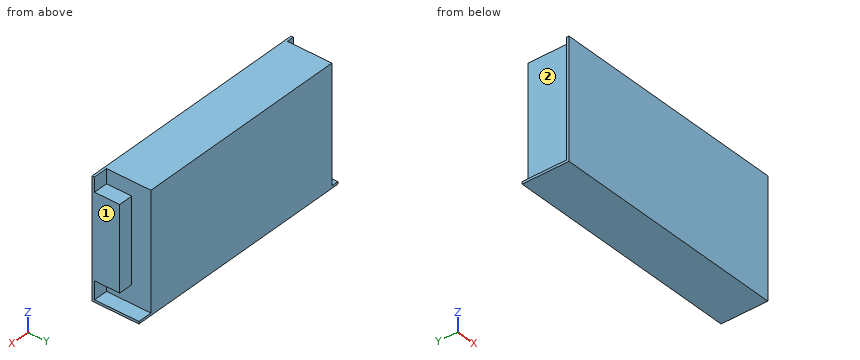
from build123d import *

# Parameters (mm, degrees)
SKETCH_1_W          = 199
SKETCH_1_H          = 99
EXTRUDE_1_DEPTH     = 39
SKETCH_2_W          = 6
SKETCH_2_H          = 97
SKETCH_2_W_2        = 12
CUT_EXTRUDE_1_DEPTH = 37
SKETCH_3_W          = 70
SKETCH_3_H          = 23
EXTRUDE_2_DEPTH     = 12


with BuildPart() as part:
    # Эскиз1 → Бобышка-Вытянуть1 (new body)
    with BuildSketch(Plane(origin=(0, 0, 0), x_dir=(1, 0, 0), z_dir=(0, 1, 0))):
        with Locations((99.5, 49.5)):
            Rectangle(SKETCH_1_W, SKETCH_1_H)
    extrude(amount=EXTRUDE_1_DEPTH)

    # Эскиз2 → Вырез-Вытянуть1 (cut)
    with BuildSketch(Plane(origin=(0, 39, 0), x_dir=(1, 0, 0), z_dir=(0, 1, 0))):
        with Locations((3, 48.5)):
            Rectangle(SKETCH_2_W, SKETCH_2_H)
        with Locations((193, 48.5)):
            Rectangle(SKETCH_2_W_2, SKETCH_2_H)
    extrude(amount=-CUT_EXTRUDE_1_DEPTH, mode=Mode.SUBTRACT)

    # Эскиз3 → Бобышка-Вытянуть2 (add)
    with BuildSketch(Plane(origin=(187, 0, 0), x_dir=(0, 0, -1), z_dir=(1, 0, 0))):
        with Locations((47, 11.5)):
            Rectangle(SKETCH_3_W, SKETCH_3_H)
    extrude(amount=EXTRUDE_2_DEPTH)


solid = part.part
Verification items for the finished model (mm, model axes). Face numbers are marked on the shaded views. A direction names the side the tool comes from. Round coordinates to 2 decimals unless told otherwise and drop trailing zeros. Loops run counter-clockwise (first coordinate to the right, second up) from the corner with the lowest first, then second, coordinate; pieces in that order, holes last. Notation, with made-up numbers: (3.5, 55) - (42.5, 55) arc R18 cw to (42.5, 62) - close; hole circle Ø5 at (-22, 0.25). An arc over 180 degrees is marked (long way). Answer in a Markdown table with one row per item. Add a question column.
Q1. Gauge pin test, flat ends, axial feed: pin 1 (13 mm diameter, centred on x = 190.5, y = 24, fed in from +Z); pin 2 (3.5 mm diameter, centred on x = 190.5, z = -91, fed in from +Y); pin 3 (9.5 mm diameter, centred on x = 192, y = 17, fed in from +Z); pin 4 (12 mm diameter, centred on y = 33.5, z = -33.5, fed in from +X). Record the tip position at first contact, or that the pin passes through.
Q2. Section check A-A on y = 6. Enter the section's corners in (x, z).
Q3. Tool access check on the marked faces 1 and 2. Record the directions out of +Z, -Z, +X, -X, +Y, -Y that give a thin tool (end or side, any length) a straight path to the whole face; none if there is none.
Q4. Material ranges on line 1 (X direction, y = 26.5, z = -7); line 2 (X direction, y = 17, z = -70), recorded low to high.
Q5. Section check C-C on y = 26.5. Enter the section's corners in (x, z), plus the area to 3 significant figures.
Q6. Section check B-B on z = -26.5. Enter the section's corners in (x, y).
Found:
| question | item | result |
|---|---|---|
| 1 | pin 1 | stops at z = 0 |
| 1 | pin 2 | stops at y = 2 |
| 1 | pin 3 | stops at z = -12 |
| 1 | pin 4 | stops at x = 187 |
| 2 | outline | (0, -99) - (199, -99) - (199, -97) - (187, -97) - (187, -82) - (199, -82) - (199, -12) - (187, -12) - (187, 0) - (6, 0) - (6, -97) - (0, -97) - close |
| 3 | face 1 | +Z, -Z, +X, +Y, -Y |
| 3 | face 2 | +Z, -X, +Y |
| 4 | line 1 | x = 6 to 187 |
| 4 | line 2 | x = 6 to 199 |
| 5 | outline | (0, -99) - (199, -99) - (199, -97) - (187, -97) - (187, 0) - (6, 0) - (6, -97) - (0, -97) - close |
| 5 | area | 18,000 mm² |
| 6 | outline | (0, 0) - (199, 0) - (199, 23) - (187, 23) - (187, 39) - (6, 39) - (6, 2) - (0, 2) - close |
